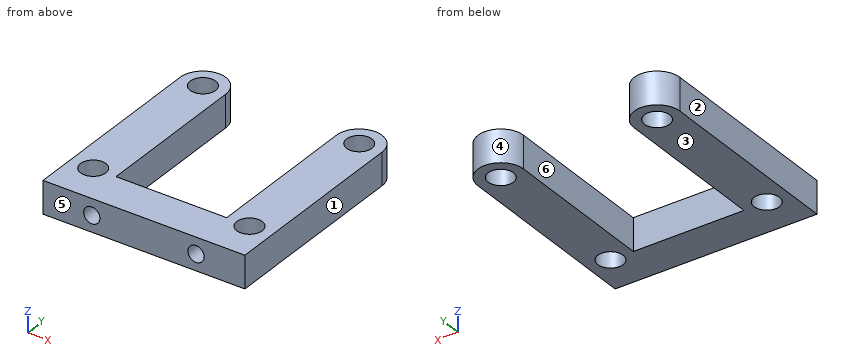
```python
from build123d import *

# Parameters (mm, degrees)
SKETCH1_R           = 1.95
BOSS_EXTRUDE1_DEPTH = 5
SKETCH4_R           = 1.25
CUT_EXTRUDE3_DEPTH  = 5.5


with BuildPart() as part:
    # Sketch1 → Boss-Extrude1 (new body)
    with BuildSketch(Plane.XY):
        with BuildLine():
            ThreePointArc((-8.5, 12), (-12, 15.5), (-15.5, 12))
            Line((-15.5, 12), (-15.5, -12))
            Line((-15.5, -12), (-15.5, -12.97105896))
            Line((-15.5, -12.97105896), (-15.5, -18))
            Line((-15.5, -18), (0, -18))
            Line((0, -18), (15.5, -18))
            Line((15.5, -18), (15.5, -12))
            Line((15.5, -12), (15.5, 12))
            ThreePointArc((15.5, 12), (12, 15.5), (8.5, 12))
            Line((8.5, 12), (8.5, -12))
            Line((8.5, -12), (0, -12))
            Line((0, -12), (-8.5, -12))
            Line((-8.5, -12), (-8.5, 12))
        make_face()
        with Locations((-12, -12)):
            Circle(SKETCH1_R, mode=Mode.SUBTRACT)
        with Locations((12, -12)):
            Circle(SKETCH1_R, mode=Mode.SUBTRACT)
        with Locations((-12, 12)):
            Circle(SKETCH1_R, mode=Mode.SUBTRACT)
        with Locations((12, 12)):
            Circle(SKETCH1_R, mode=Mode.SUBTRACT)
    extrude(amount=BOSS_EXTRUDE1_DEPTH)

    # Sketch4 → Cut-Extrude3 (cut)
    with BuildSketch(Plane.XZ.offset(18)):
        with Locations((-8, 2.5)):
            Circle(SKETCH4_R)
        with Locations((8, 2.5)):
            Circle(SKETCH4_R)
    extrude(amount=-CUT_EXTRUDE3_DEPTH, mode=Mode.SUBTRACT)


solid = part.part
```
Build history of the part. All positions in model axes, mm. Face numbers are marked on the shaded views. A direction names the side the tool comes from. Give positions to 0.01 mm unless a question says otherwise; leave off trailing zeros. Loops run counter-clockwise (first coordinate to the right, second up) from the corner with the lowest first, then second, coordinate; pieces in that order, holes last.
1) Band-saw the part on D-D on y = -13.5. List the corners of the cut face in (x, z).
Values follow:
outline: (-15.5, 0) - (-13.25, 0) - (-13.25, 5) - (-15.5, 5) - close; (-10.75, 0) - (10.75, 0) - (10.75, 5) - (-10.75, 5) - close; (13.25, 0) - (15.5, 0) - (15.5, 5) - (13.25, 5) - close; hole circle Ø2.5 at (-8, 2.5); hole circle Ø2.5 at (8, 2.5)
2) Probe line 1 along Y through (x, z) = (12, 3.9); line 2 along X through (y, z) = (13.5, 4.8); line 3 along X through (y, z) = (-0.5, 0.6). List the from-to ranges inside material, lowest first.
Values follow:
line 1: y = -18 to -13.95, -10.05 to 10.05, 13.95 to 15.5
line 2: x = -15.16 to -13.25, -10.75 to -8.84, 8.84 to 10.75, 13.25 to 15.16
line 3: x = -15.5 to -8.5, 8.5 to 15.5
3) Two-plate mould, pull along X, no slides. Class the marked faces 1, 2, 3 and 4: released by +X, released by -X, zero draft, split by the parting line, or undercut.
Values follow:
face 1: released by +X
face 2: released by -X
face 3: zero draft
face 4: undercut
4) Band-saw the part on B-B on x = -12. List the corners of the cut face in (y, z), then the cut area to 4 significant figures.
Values follow:
outline: (-18, 0) - (-13.95, 0) - (-13.95, 5) - (-18, 5) - close; (-10.05, 0) - (10.05, 0) - (10.05, 5) - (-10.05, 5) - close; (13.95, 0) - (15.5, 0) - (15.5, 5) - (13.95, 5) - close
area: 128.5 mm2
5) 3-axis set-ups, long thin cutter, end or side, ignore diameter. For the marked faces 5 and 6: which of +Z, -Z, +X, -X, +Y, -Y reach the whole face in a straight line?
Values follow:
face 5: +Z, -Z, +X, -X, -Y
face 6: +Z, -Z, +Y
6) Drop flat-ended pins along their axis: P1, Ø2.5, axis at x = -1.5, z = 2.5, coming from the +Y side; P2, Ø1.5, axis at x = 8, z = 2.5, coming from the -Y side. Give the stop position or say it passes through.
Values follow:
P1: stops at y = -12
P2: stops at y = -12.5
7) Band-saw the part on A-A on y = -6.5. List the corners of the cut face in (x, z), then the cut area to 3 significant figures.
Values follow:
outline: (-15.5, 0) - (-8.5, 0) - (-8.5, 5) - (-15.5, 5) - close; (8.5, 0) - (15.5, 0) - (15.5, 5) - (8.5, 5) - close
area: 70.0 mm2
8) Band-saw the part on C-C on z = 0.7. List the corners of the cut face in (x, y), then the cut area to 3 significant figures.
Values follow:
outline: (-15.5, -18) - (15.5, -18) - (15.5, 12) arc R3.5 ccw to (8.5, 12) - (8.5, -12) - (-8.5, -12) - (-8.5, 12) arc R3.5 ccw to (-15.5, 12) - close; hole circle Ø3.9 at (-12, -12); hole circle Ø3.9 at (-12, 12); hole circle Ø3.9 at (12, -12); hole circle Ø3.9 at (12, 12)
area: 513 mm2
